Geometry: see drawing. Coordinates: mm, zero at the bounding-box minimum. Coordinates: 2 decimals unless noted, no trailing zeros. Order: outer loops, then holes, each group sorted by start corner. A loop starts at its lowest first (then second) coordinate and runs counter-clockwise, first axis right, second up. Notation, with made-up numbers: M 34.5,45.5 L 80.5,45.5 A24 cw 80.5,61.5 Z; hole C 23,-33.5 d7. An arc over 180 degrees is marked long. Answer in a Markdown table with one row per item.
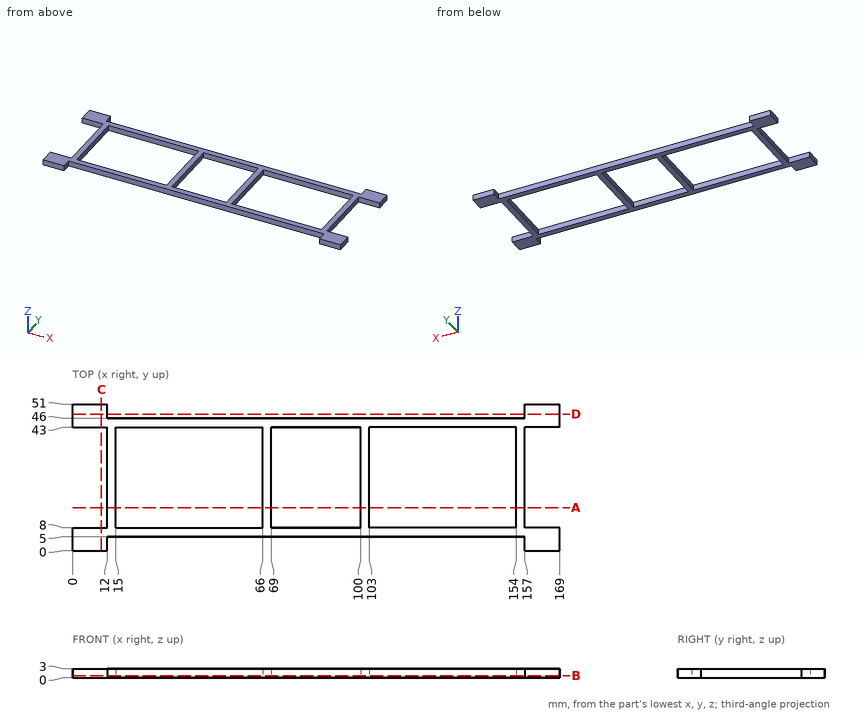
1) Cut plane B-B, the plane z = 0.65. State how many separate pieces and enclosed holes the cut face has, and give its area (3 significant figures).
Resolved:
| item | result |
|---|---|
| separate pieces | 1 |
| enclosed holes | 3 |
| area | 1,670 mm2 |
2) Contact query for flat-ended pins moving along their axis: pin 1 (1.5 mm diameter, centred on y = 20, z = 0.5, fed in from -X); pin 2 (1.5 mm diameter, centred on y = 18.5, z = 2, fed in from +X); pin 3 (1.5 mm diameter, centred on x = 17.5, y = 28.5, fed in from -Z); pin 4 (0.9 mm diameter, centred on x = 29.5, z = 1.5, fed in from +Y). Output: stop coordinate, or through.
Resolved:
| item | result |
|---|---|
| pin 1 | stops at x = 12 |
| pin 2 | stops at x = 157 |
| pin 3 | passes through |
| pin 4 | stops at y = 46 |
3) Material intervals for probe 1 along X at (y, z) = (16, 0.9); probe 2 along Y at (x, z) = (160.5, 1.45); probe 3 along Y at (x, z) = (113, 0.55), sorted ascending.
Resolved:
| item | result |
|---|---|
| probe 1 | x = 12 to 15, 66 to 69, 100 to 103, 154 to 157 |
| probe 2 | y = 0 to 8, 43 to 51 |
| probe 3 | y = 5 to 8, 43 to 46 |
4) Cut plane D-D, the plane y = 47.5. Output: boundary loops of the cut face in (x, z).
Resolved:
| item | result |
|---|---|
| outline | M 0,0 L 12,0 L 12,3 L 0,3 Z; M 157,0 L 169,0 L 169,3 L 157,3 Z |
5) Cut plane C-C, the plane x = 10. Output: boundary loops of the cut face in (y, z), and give its area (3 significant figures).
Resolved:
| item | result |
|---|---|
| outline | M 0,0 L 8,0 L 8,3 L 0,3 Z; M 43,0 L 51,0 L 51,3 L 43,3 Z |
| area | 48.0 mm2 |
6) Cut plane A-A, the plane y = 15. Output: boundary loops of the cut face in (x, z), and give its area (3 significant figures).
Resolved:
| item | result |
|---|---|
| outline | M 12,0 L 15,0 L 15,3 L 12,3 Z; M 66,0 L 69,0 L 69,3 L 66,3 Z; M 100,0 L 103,0 L 103,3 L 100,3 Z; M 154,0 L 157,0 L 157,3 L 154,3 Z |
| area | 36.0 mm2 |
